Autodesk Inventor part; units mm, degrees
ref_plane "YZ Plane" through (0, 0, 0) normal (1, 0, 0) x (0, 1, 0)
ref_plane "XZ Plane" through (0, 0, 0) normal (0, 1, 0) x (-1, 0, 0)
ref_plane "XY Plane" through (0, 0, 0) normal (0, 0, 1) x (1, 0, 0)
sketch "Sketch1" plane through (0, 0, 0) normal (0, 1, 0) x (-1, 0, 0)
  circle A0 centre (0, 0) radius 44.45
  circle A1 centre (0, -41.275) radius 1.6
  circle A2 centre (35.7452, -20.6375) radius 1.6
  circle A3 centre (-35.7452, -20.6375) radius 1.6
  circle A4 centre (0, 41.275) radius 1.6
  circle A5 centre (35.7452, 20.6375) radius 1.6
  circle A6 centre (-35.7452, 20.6375) radius 1.6
  circle A7 centre (-12.7279, -12.7279) radius 15.4558
extrude "Extrusion2" add sketch "Sketch1" along normal blind 13
sketch "Sketch2" plane through (0, 13, 0) normal (0, 1, 0) x (1, 0, 0)
  circle A0 centre (12.7279, 12.7279) radius 15.4558
  circle A1 centre (12.7279, 12.7279) radius 20
  circle A2 centre (0, 0) radius 44.45
  dimension "d27" = 40
extrude "Extrusion3" cut sketch "Sketch2" against normal blind 10 contours A2
properties part number "Potting_Jig_External"
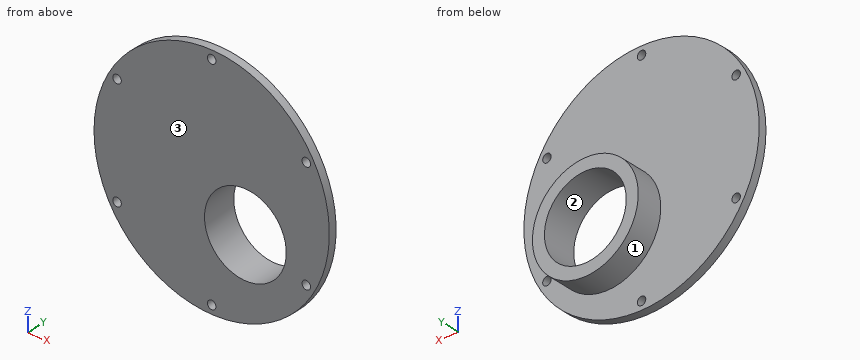
Model file for the job. Use its own axes, mm. Face numbers are marked on the shaded views. Coordinates: 2 decimals unless noted, no trailing zeros. Write each loop counter-clockwise with the first axis right and the second up, starting at its lowest first coordinate (ties: lowest second). Pieces come first, ordered by that corner, then holes. Notation, with made-up numbers: (89, -14.75) - (114, -14.75) arc R13 ccw to (114, 4.25) - close; hole circle Ø8 at (18.25, -18). An arc over 180 degrees is marked (long way). Use a Markdown table: item, result. Add a question column.
Item 1: Drop flat-ended pins along their axis: pin 1 (4 mm diameter, centred on x = 0, z = -41.275, fed in from +Y); pin 2 (6 mm diameter, centred on x = 8, y = 10, fed in from -Z); pin 3 (5 mm diameter, centred on x = 14, y = 8.5, fed in from +Z); pin 4 (1.9 mm diameter, centred on x = 35.75, z = 20.64, fed in from -Y). Give the stop position or say it passes through.
Item 2: Band-saw the part on C-C, the plane y = 1.25. Give the number of separate pieces and of enclosed holes in the cut face, and give its area (3 significant figures).
Item 3: Band-saw the part on A-A, the plane z = -14.5. Write the cut outline in (x, y), and give its area (3 significant figures).
Item 4: Two-plate mould, pull along X, no slides. Class the marked faces 1, 2 and 3: pulls with the +X half, pulls with the -X half, needs draft (parallel to the pull), parting line crosses it, or undercut.
Item 5: Drill centre lines: line 1 along Z through (x, y) = (0, 1.25) (3 decimals); line 2 along Y through (x, z) = (-27, -2); line 3 along X through (y, z) = (3.5, 1). Where is each one in solid material? Low to high.
Item 6: Band-saw the part on B-B, the plane x = 3.5. Write the cut outline in (y, z), and give its area (3 significant figures).
Item 7: Band-saw the part on D-D, the plane y = 10.5. Write the cut outline in (x, z).
A:
| question | item | result |
|---|---|---|
| 1 | pin 1 | stops at y = 3 |
| 1 | pin 2 | stops at z = -32.65 |
| 1 | pin 3 | stops at z = 7.27 |
| 1 | pin 4 | passes through |
| 2 | separate pieces | 1 |
| 2 | enclosed holes | 7 |
| 2 | area | 5,410 mm² |
| 3 | outline | (-42.02, 0) - (-2.63, 0) - (-2.63, 13) - (-7.19, 13) - (-7.19, 3) - (-42.02, 3) - close; (28.08, 0) - (42.02, 0) - (42.02, 3) - (32.65, 3) - (32.65, 13) - (28.08, 13) - close |
| 3 | area | 251 mm² |
| 4 | face 1 | parting line crosses it |
| 4 | face 2 | undercut |
| 4 | face 3 | needs draft |
| 5 | line 1 | z = -44.45 to -42.875, -39.675 to -21.496, -3.96 to 39.675, 42.875 to 44.45 |
| 5 | line 2 | y = 0 to 3 |
| 5 | line 3 | x = -1.82 to 5.63, 19.83 to 27.27 |
| 6 | outline | (0, -44.31) - (3, -44.31) - (3, -30.47) - (13, -30.47) - (13, -25.13) - (0, -25.13) - close; (0, -0.33) - (13, -0.33) - (13, 5.02) - (3, 5.02) - (3, 44.31) - (0, 44.31) - close |
| 6 | area | 298 mm² |
| 7 | outline | circle Ø40 at (12.73, -12.73); hole circle Ø30.91 at (12.73, -12.73) |
